The figure shows three views and two pictorial views of one solid part (mm, origin at its lowest corner). Answer the questions. Coordinates: 2 decimals unless noted, no trailing zeros. Order: outer loops, then holes, each group sorted by start corner. A loop starts at its lowest first (then second) coordinate and runs counter-clockwise, first axis right, second up. Notation, with made-up numbers: M -30.75,26.25 L -10.75,26.25 A27 ccw -10.75,63.25 Z; hole C -28.75,13 d9. An arc over 180 degrees is marked long. Answer in a Markdown table with one row per item. Add a question column.
Item 1: Consider line 1 (X direction, y = 26, z = 57); line 2 (Z direction, x = 50, y = 22); line 3 (Z direction, x = 44, y = 15). Determine where each line is inside the solid, lowest interval first. Write a range as from..to.
Item 2: The part is cut by section D-D (z = 131). Write down the section's boundary in (x, y).
Item 3: The part is cut by section C-C (y = 8). Write down the section's boundary in (x, z).
Item 4: The part is cut by section A-A (z = 57.15). Write down the section's boundary in (x, y).
Item 5: The part is cut by section B-B (x = 838.2). Write down the section's boundary in (y, z).
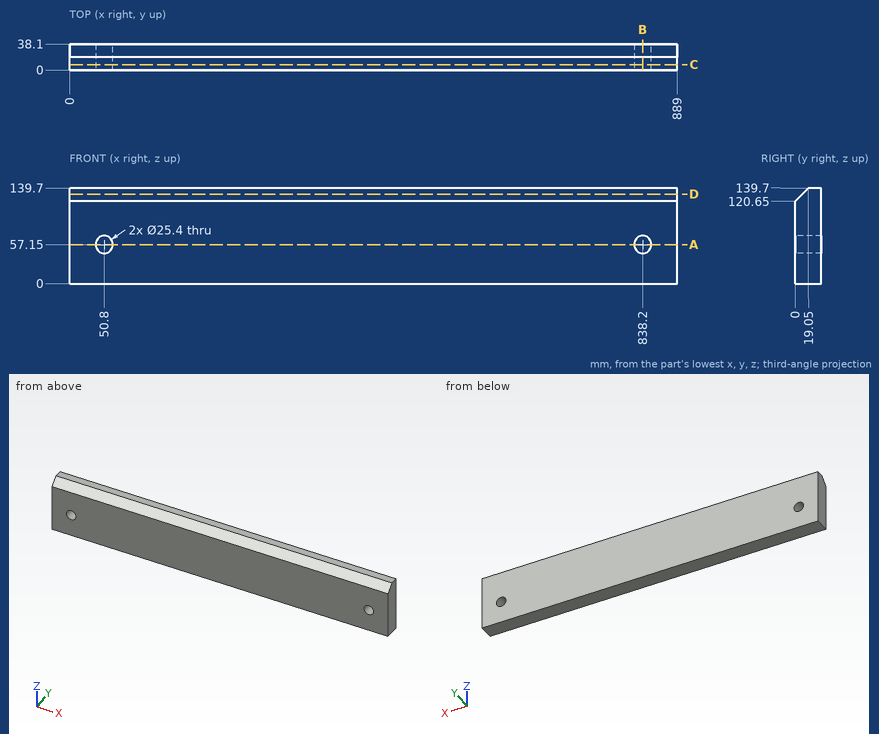
Reply:
| question | item | result |
|---|---|---|
| 1 | line 1 | x = 0..38.1, 63.5..825.5, 850.9..889 |
| 1 | line 2 | z = 0..44.48, 69.82..139.7 |
| 1 | line 3 | z = 0..46.42, 67.88..135.65 |
| 2 | outline | M 0,10.35 L 889,10.35 L 889,38.1 L 0,38.1 Z |
| 3 | outline | M 0,0 L 889,0 L 889,128.65 L 0,128.65 Z; hole C 50.8,57.15 d25.4; hole C 838.2,57.15 d25.4 |
| 4 | outline | M 0,0 L 38.1,0 L 38.1,38.1 L 0,38.1 Z; M 63.5,0 L 825.5,0 L 825.5,38.1 L 63.5,38.1 Z; M 850.9,0 L 889,0 L 889,38.1 L 850.9,38.1 Z |
| 5 | outline | M 0,0 L 38.1,0 L 38.1,44.45 L 0,44.45 Z; M 0,69.85 L 38.1,69.85 L 38.1,139.7 L 19.05,139.7 L 0,120.65 Z |
